from build123d import *

# Parameters (mm, degrees)
SKETCH_1_W          = 24
SKETCH_1_H          = 27
EXTRUDE_1_DEPTH     = 10
SKETCH_4_R          = 2.1
CUT_EXTRUDE_2_DEPTH = 37.013519789
SKETCH_2_R          = 11
EXTRUDE_2_DEPTH     = 4
SKETCH_5_R          = 7.5
EXTRUDE_3_DEPTH     = 3
SKETCH_6_R          = 5.75
EXTRUDE_4_DEPTH     = 0.5
SKETCH_7_R          = 6
EXTRUDE_5_DEPTH     = 11.5
SKETCH_8_R          = 5.75
EXTRUDE_6_DEPTH     = 1.1
SKETCH_9_R          = 6
EXTRUDE_7_DEPTH     = 2
CHAMFER_1_SIZE      = 0.5
CHAMFER_2_SIZE      = 2


with BuildPart() as part:
    # 草图1 → 凸台-拉伸1 (new body)
    with BuildSketch(Plane.XY):
        Rectangle(SKETCH_1_W, SKETCH_1_H)
    extrude(amount=EXTRUDE_1_DEPTH)

    # 草图4 → 切除-拉伸2 (cut)
    with BuildSketch(Plane(origin=(0, 13.5, 0), x_dir=(1, 0, 0), z_dir=(0, 1, 0))):
        with Locations(Location((-8, -5, 0), (0, 0, 270))):
            Circle(SKETCH_4_R)
        with Locations(Location((8, -5, 0), (0, 0, 270))):
            Circle(SKETCH_4_R)
    extrude(amount=-CUT_EXTRUDE_2_DEPTH, mode=Mode.SUBTRACT)

    # 草图2 → 凸台-拉伸2 (add)
    with BuildSketch(Plane.XY):
        Circle(SKETCH_2_R)
    extrude(amount=-EXTRUDE_2_DEPTH)

    # 草图5 → 凸台-拉伸3 (add)
    with BuildSketch(Plane(origin=(0, 0, -4), x_dir=(-1, 0, 0), z_dir=(0, 0, -1))):
        with Locations(Location((0, 0, 0), (0, 0, 180))):
            Circle(SKETCH_5_R)
    extrude(amount=EXTRUDE_3_DEPTH)

    # 草图6 → 凸台-拉伸4 (add)
    with BuildSketch(Plane(origin=(0, 0, -7), x_dir=(-1, 0, 0), z_dir=(0, 0, -1))):
        Circle(SKETCH_6_R)
    extrude(amount=EXTRUDE_4_DEPTH)

    # 草图7 → 凸台-拉伸5 (add)
    with BuildSketch(Plane(origin=(0, 0, -7.5), x_dir=(-1, 0, 0), z_dir=(0, 0, -1))):
        Circle(SKETCH_7_R)
    extrude(amount=EXTRUDE_5_DEPTH)

    # 草图8 → 凸台-拉伸6 (add)
    with BuildSketch(Plane(origin=(0, 0, -19), x_dir=(-1, 0, 0), z_dir=(0, 0, -1))):
        Circle(SKETCH_8_R)
    extrude(amount=EXTRUDE_6_DEPTH)

    # 草图9 → 凸台-拉伸7 (add)
    with BuildSketch(Plane(origin=(0, 0, -20.1), x_dir=(-1, 0, 0), z_dir=(0, 0, -1))):
        Circle(SKETCH_9_R)
    extrude(amount=EXTRUDE_7_DEPTH)

    # 倒角1
    chamfer_1_edges = [part.edges().sort_by_distance(p)[0] for p in [
        (6, 0, -22.1),
    ]]
    chamfer(chamfer_1_edges, length=CHAMFER_1_SIZE)

    # 倒角2
    chamfer_2_edges = [part.edges().sort_by_distance(p)[0] for p in [
        (-12, 0, 10),
    ]]
    chamfer(chamfer_2_edges, length=CHAMFER_2_SIZE)


solid = part.part
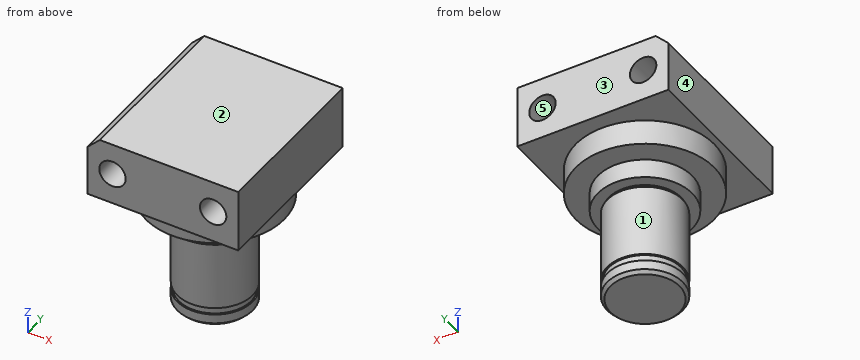
Here's how the part is built. I have some questions about the finished solid (model axes, mm). Face numbers are marked on the shaded views. A direction names the side the tool comes from. Give positions to 0.01 mm unless a question says otherwise; leave off trailing zeros. Loops run counter-clockwise (first coordinate to the right, second up) from the corner with the lowest first, then second, coordinate; pieces in that order, holes last. Notation, with made-up numbers: (50.25, 82) -> (70.25, 82) arc R28 ccw to (70.25, 116) -> close; hole circle Ø8 at (33.5, 27.25). An arc over 180 degrees is marked (long way). Answer as a JSON object with one key per item and string values. Group by question number.
Item 1: Will these pins go through, and if not, where does the flat tip stop? pin 1 (6 mm diameter, centred on x = -8.5, y = 1, fed in from -Z); pin 2 (2.5 mm diameter, centred on x = -8, z = 5, fed in from +Y); pin 3 (12 mm diameter, centred on x = -8.5, y = 2, fed in from -Z); pin 4 (5 mm diameter, centred on x = 6.5, z = -17.5, fed in from +Y).
Item 2: Imagine slicing it at A-A on y = 0. Give the number of separate pieces and of enclosed holes in the cut face, then the cut area to 3 significant figures.
Item 3: On a 3-axis mill with a long thin cutter (end or side, diameter ignored), from which of +Z, -Z, +X, -X, +Y, -Y can I reach the whole of each face in a straight line? I mean the marked faces 1 and 2. Say none if no direction works.
Item 4: Imagine slicing it at B-B on x = -8. Write out the boundary of the cut face in (y, z).
Item 5: I need wall thicknesses on L1, parallel to X at y = 4.25, z = 5; L2, parallel to X at y = -0.75, z = 6; L3, parallel to Z at x = 5.5, y = 4.5. Which ranges of each line are inside material? Lowest first, please.
Item 6: Thinking about a two-plate mould opening in X: for the marked faces 3, 4 and 5, which applies, pulls with the +X half, pulls with the -X half, needs draft (parallel to the pull), parting line crosses it, or undercut?
Item 7: Imagine slicing it at D-D on y = -11.5. Write out the boundary of the cut face in (x, z), then the cut area to 3 significant figures.
Answer list:
{
 "1": {"pin 1": "stops at z = -22.04", "pin 2": "passes through", "pin 3": "stops at z = -22.1", "pin 4": "stops at y = 4.47"},
 "2": {"separate pieces": "1", "enclosed holes": "2", "area": "523 mm2"},
 "3": {"face 1": "-Z", "face 2": "+Z, +X, -X, +Y, -Y"},
 "4": {"outline": "(-13.5, 0) -> (-7.55, 0) -> (-7.55, -4) -> (7.55, -4) -> (7.55, 0) -> (13.5, 0) -> (13.5, 2.9) -> (-13.5, 2.9) -> close; (-13.5, 7.1) -> (13.5, 7.1) -> (13.5, 10) -> (-13.5, 10) -> close"},
 "5": {"L1": "x = -12 to -10.1, -5.9 to 5.9, 10.1 to 12", "L2": "x = -12 to -9.85, -6.15 to 6.15, 9.85 to 12", "L3": "z = -7 to 10"},
 "6": {"face 3": "needs draft", "face 4": "pulls with the -X half", "face 5": "undercut"},
 "7": {"outline": "(-12, 0) -> (12, 0) -> (12, 10) -> (-10, 10) -> (-12, 8) -> close; hole circle Ø4.2 at (-8, 5); hole circle Ø4.2 at (8, 5)", "area": "210 mm2"}
}
